CAD build for the part. Positions are in the model's coordinates, mm. Face numbers are marked on the shaded views. A direction names the side the tool comes from. Coordinates: 2 decimals unless noted, no trailing zeros. Answer as a JSON object with one key per item and string values. Group by question number.
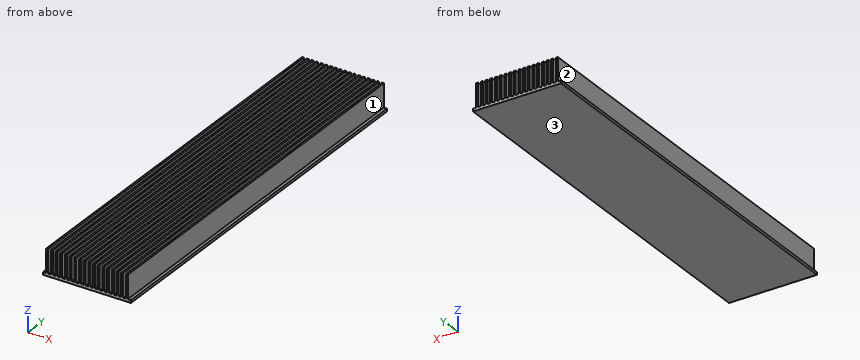
from build123d import *

# Parameters (mm, degrees)
F0_W     = 2.5
F0_H     = 30
F1_DEPTH = 500


with BuildPart() as f1:
    # F0 (on Front) → F1 (new body)
    with BuildSketch(Plane.XZ):
        Polygon((-56.25, 0), (0, 0), (56.25, 0), (56.25, 3.5), (52.25, 3.5), (52.25, 33.5), (49.75, 33.5), (49.75, 3.5), (46.25, 3.5), (43.75, 3.5), (40.25, 3.5), (37.75, 3.5), (34.25, 3.5), (31.75, 3.5), (28.25, 3.5), (25.75, 3.5), (22.25, 3.5), (19.75, 3.5), (16.25, 3.5), (13.75, 3.5), (10.25, 3.5), (7.75, 3.5), (4.25, 3.5), (1.75, 3.5), (-1.75, 3.5), (-4.25, 3.5), (-7.75, 3.5), (-10.25, 3.5), (-13.75, 3.5), (-16.25, 3.5), (-19.75, 3.5), (-22.25, 3.5), (-25.75, 3.5), (-28.25, 3.5), (-31.75, 3.5), (-34.25, 3.5), (-37.75, 3.5), (-40.25, 3.5), (-43.75, 3.5), (-46.25, 3.5), (-49.75, 3.5), (-52.25, 3.5), (-56.25, 3.5), align=None)
        with Locations((-51, 18.5)):
            Rectangle(F0_W, F0_H)
        with Locations((-45, 18.5)):
            Rectangle(F0_W, F0_H)
        with Locations((45, 18.5)):
            Rectangle(F0_W, F0_H)
        with Locations((-39, 18.5)):
            Rectangle(F0_W, F0_H)
        with Locations((39, 18.5)):
            Rectangle(F0_W, F0_H)
        with Locations((-33, 18.5)):
            Rectangle(F0_W, F0_H)
        with Locations((33, 18.5)):
            Rectangle(F0_W, F0_H)
        with Locations((-27, 18.5)):
            Rectangle(F0_W, F0_H)
        with Locations((27, 18.5)):
            Rectangle(F0_W, F0_H)
        with Locations((-21, 18.5)):
            Rectangle(F0_W, F0_H)
        with Locations((21, 18.5)):
            Rectangle(F0_W, F0_H)
        with Locations((-15, 18.5)):
            Rectangle(F0_W, F0_H)
        with Locations((15, 18.5)):
            Rectangle(F0_W, F0_H)
        with Locations((-9, 18.5)):
            Rectangle(F0_W, F0_H)
        with Locations((9, 18.5)):
            Rectangle(F0_W, F0_H)
        with Locations((-3, 18.5)):
            Rectangle(F0_W, F0_H)
        with Locations((3, 18.5)):
            Rectangle(F0_W, F0_H)
    extrude(amount=F1_DEPTH)


solid = f1.part
Item 1: Band-saw the part on A-A, the plane z = 13. Count the separate pieces of the cut face and the enclosed holes in it, and give its area (3 significant figures).
Item 2: 3-axis set-ups, long thin cutter, end or side, ignore diameter. For the marked faces 1, 2 and 3: which of +Z, -Z, +X, -X, +Y, -Y reach the whole face in a straight line?
Item 3: Drill centre line: L1, parallel to Z at x = 31, y = -145.5. Where is it in solid material? Low to high.
Item 4: Flat gauge pins, fed straight in: P1, Ø15, axis at y = -351.5, z = 14.5, coming from the +X side; P2, Ø2, axis at x = 30, y = -210, coming from the +Z side; P3, Ø9, axis at y = -270, z = 22, coming from the -X side. Where does each tip first touch, or does it go through?
Reply:
{
 "1": {"separate pieces": "18", "enclosed holes": "0", "area": "22,500 mm²"},
 "2": {"face 1": "+Z, +X, +Y, -Y", "face 2": "+Z, -X, +Y, -Y", "face 3": "-Z, +X, -X, +Y, -Y"},
 "3": {"L1": "0 to 3.5"},
 "4": {"P1": "x = 52.25", "P2": "z = 3.5", "P3": "x = -52.25"}
}
